The listing builds one solid part. Answer for the finished solid, in the listing's coordinates (mm). Round coordinates to 2 decimals unless told otherwise and drop trailing zeros. Loops run counter-clockwise (first coordinate to the right, second up) from the corner with the lowest first, then second, coordinate; pieces in that order, holes last. Notation, with made-up numbers: M 6,23.5 L 53,23.5 A34 ccw 53,59.5 Z; hole C 5,62.5 d8. An arc over 180 degrees is marked long. Answer as a JSON object with one key per item and string values.
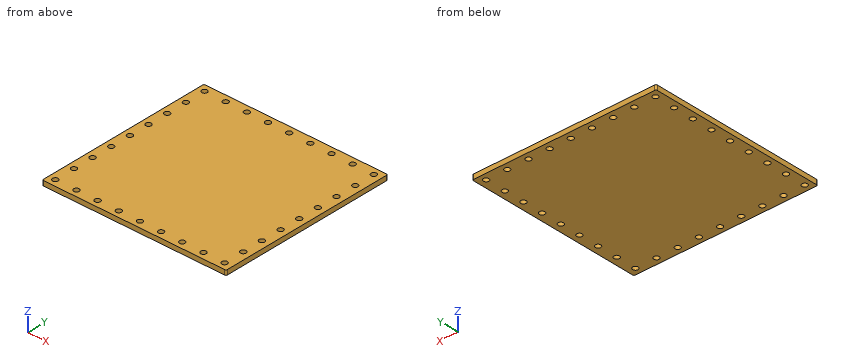
Autodesk Inventor part; units mm, degrees
ref_plane "YZ Plane" through (0, 0, 0) normal (1, 0, 0) x (0, 1, 0)
ref_plane "XZ Plane" through (0, 0, 0) normal (0, 1, 0) x (-1, 0, 0)
ref_plane "XY Plane" through (0, 0, 0) normal (0, 0, 1) x (1, 0, 0)
ref_plane "РабПлоскость1" through (0, 0, 0) normal (0, 0, 1) x (1, 0, 0)
sketch "Эскиз1" plane through (0, 0, 0) normal (0, 0, 1) x (1, 0, 0)
  line L0 (-134.636, 128) -> (-134.636, -128)
  arc A0 (-134.636, -128) -> (-132.636, -130) centre (-132.636, -128) ccw
  line L1 (-132.636, -130) -> (132.636, -130)
  arc A1 (132.636, -130) -> (134.636, -128) centre (132.636, -128) ccw
  line L2 (134.636, -128) -> (134.636, 128)
  arc A2 (134.636, 128) -> (132.636, 130) centre (132.636, 128) ccw
  line L3 (132.636, 130) -> (-132.636, 130)
  arc A3 (-132.636, 130) -> (-134.636, 128) centre (-132.636, 128) ccw
  circle A4 centre (-124.636, 120) radius 4
  circle A5 centre (-124.636, 60) radius 4
  circle A6 centre (-124.636, 0) radius 4
  circle A7 centre (-124.636, -60) radius 4
  circle A8 centre (-124.636, -120) radius 4
  circle A9 centre (-93.636, -120) radius 4
  circle A10 centre (-62.636, -120) radius 4
  circle A11 centre (-31.636, -120) radius 4
  circle A12 centre (-0.636, -120) radius 4
  circle A13 centre (30.364, -120) radius 4
  circle A14 centre (61.364, -120) radius 4
  circle A15 centre (92.364, -120) radius 4
  circle A16 centre (123.364, 90) radius 4
  circle A17 centre (123.364, 60) radius 4
  circle A18 centre (123.364, 30) radius 4
  circle A19 centre (123.364, 0) radius 4
  circle A20 centre (123.364, -30) radius 4
  circle A21 centre (123.364, -60) radius 4
  circle A22 centre (123.364, -90) radius 4
  circle A23 centre (123.364, -120) radius 4
  circle A24 centre (123.364, 120) radius 4
  circle A25 centre (92.364, 120) radius 4
  circle A26 centre (61.364, 120) radius 4
  circle A27 centre (30.364, 120) radius 4
  circle A28 centre (-0.636, 120) radius 4
  circle A29 centre (-31.636, 120) radius 4
  circle A30 centre (-62.636, 120) radius 4
  circle A31 centre (-93.636, 120) radius 4
  circle A32 centre (-124.636, -90) radius 4
  circle A33 centre (-124.636, -30) radius 4
  circle A34 centre (-124.636, 30) radius 4
  circle A35 centre (-124.636, 90) radius 4
  line L4 (115.364, 110) -> (115.364, -110)
  line L5 (115.364, -110) -> (-114.636, -110)
  line L6 (-114.636, -110) -> (-114.636, 110)
  line L7 (-114.636, 110) -> (115.364, 110)
  point P0 (0, 0)
extrude "Выдавливание1" add sketch "Эскиз1" along normal blind 7 contours A3 L3 A2 L2 A1 L1 A0 L0 | L4 L5 L6 L7
properties part number "Крышка рубашки охлаждения" material "Чугун, серый"
Item 1: The part is cut by section B-B (x = 0). Give the vertices of the cut face in (y, z), then the cut area to 3 significant figures.
Values follow:
{"outline": "M -130,0 L -123.95,0 L -123.95,7 L -130,7 Z; M -116.05,0 L 116.05,0 L 116.05,7 L -116.05,7 Z; M 123.95,0 L 130,0 L 130,7 L 123.95,7 Z", "area": "1,710 mm^2"}
Item 2: The part is cut by section A-A (y = -60). Give the vertices of the cut face in (x, z).
Values follow:
{"outline": "M -134.64,0 L -128.64,0 L -128.64,7 L -134.64,7 Z; M -120.64,0 L 119.36,0 L 119.36,7 L -120.64,7 Z; M 127.36,0 L 134.64,0 L 134.64,7 L 127.36,7 Z"}
Item 3: A flat-ended cylindrical pin translates along its axis: P1, Ø10.5, axis at x = -62.636, y = 120, coming from the -Z side. Find the tip coordinate at first contact, or state that the pin passes through.
Values follow:
{"P1": "z = 0"}
Item 4: The part is cut by section C-C (z = 5.5). Give the number of separate pieces and of enclosed holes in the cut face, then the cut area to 3 significant figures.
Values follow:
{"separate pieces": "1", "enclosed holes": "32", "area": "68,400 mm^2"}
Item 5: Straight lines are drawn through the part: line 1 (Y direction, x = -32, z = 4); line 2 (Y direction, x = -28, z = 6.5); line 3 (X direction, y = -3.5, z = 5). For each, find the intervals that lie inside material, in ascending order.
Values follow:
{"line 1": "-130 to -123.98, -116.02 to 116.02, 123.98 to 130", "line 2": "-130 to -121.67, -118.33 to 118.33, 121.67 to 130", "line 3": "-134.64 to -126.57, -122.7 to 121.43, 125.3 to 134.64"}
